```python
from build123d import *

# Parameters (mm, degrees)
SKETCH_1_W          = 100
SKETCH_1_H          = 40
EXTRUDE_1_DEPTH     = 2
EXTRUDE_2_DEPTH     = 2
SKETCH_4_R          = 3.5
CUT_EXTRUDE_1_DEPTH = 2


with BuildPart() as part:
    # 草图1 → 凸台-拉伸1 (new body)
    with BuildSketch(Plane(origin=(0, 0, 0), x_dir=(1, 0, 0), z_dir=(0, 1, 0))):
        with Locations((50, 20)):
            Rectangle(SKETCH_1_W, SKETCH_1_H)
    extrude(amount=EXTRUDE_1_DEPTH)

    # 草图3 → 凸台-拉伸2 (add)
    with BuildSketch(Plane.XY):
        with BuildLine():
            Line((72.5, 0), (27.5, 0))
            Line((27.5, 0), (37.539738947, 55.648838734))
            ThreePointArc((37.539738947, 55.648838734), (35.238312644, 66.663191018), (41.243617117, 76.178906306))
            Line((41.243617117, 76.178906306), (45, 97))
            Line((45, 97), (55, 97))
            Line((55, 97), (58.756382883, 76.178906306))
            ThreePointArc((58.756382883, 76.178906306), (64.761687356, 66.663191018), (62.460261053, 55.648838734))
            Line((62.460261053, 55.648838734), (72.5, 0))
        make_face()
    extrude(amount=EXTRUDE_2_DEPTH)

    # 草图4 → 切除-拉伸1 (cut)
    with BuildSketch(Plane.XY.offset(2)):
        with Locations((50, 64)):
            Circle(SKETCH_4_R)
    extrude(amount=-CUT_EXTRUDE_1_DEPTH, mode=Mode.SUBTRACT)


solid = part.part
```
Build history of the part. All positions in model axes, mm. A direction names the side the tool comes from. Give positions to 0.01 mm unless a question says otherwise; leave off trailing zeros. Loops run counter-clockwise (first coordinate to the right, second up) from the corner with the lowest first, then second, coordinate; pieces in that order, holes last. Notation, with made-up numbers: (66, -23.75) -> (112, -23.75) arc R17 cw to (112, -12.75) -> close; hole circle Ø11 at (62, 89.5). An arc over 180 degrees is marked (long way). One line per question, with ' | ' between items.
Q1. Tool access for faces 4 (the flat face through (50, 40, 0)), 5 (the cylindrical face through (64.732, 66.822, 0.986)): list every direction of +Z, -Z, +X, -X, +Y, -Y with a clear straight run to the whole face (end or side of a thin tool).
Filled sheet:
face 4: -Z, +X, -X, +Y | face 5: +Z, -Z, +X
Q2. Cut at B-B, the plane y = 64. Write the cut outline in (x, z).
Filled sheet:
outline: (35, 0) -> (46.5, 0) -> (46.5, 2) -> (35, 2) -> close; (53.5, 0) -> (65, 0) -> (65, 2) -> (53.5, 2) -> close
Q3. Drill centre lines: line 1 along Y through (x, z) = (50, 0.7); line 2 along Y through (x, z) = (18, -38). Where is each one in solid material? Low to high. Write a range as [from, to].
Filled sheet:
line 1: y = [0, 60.5], [67.5, 97] | line 2: y = [0, 2]
Q4. Cut at A-A, the plane x = 50. Write the cut outline in (y, z).
Filled sheet:
outline: (0, -40) -> (2, -40) -> (2, 0) -> (60.5, 0) -> (60.5, 2) -> (0, 2) -> close; (67.5, 0) -> (97, 0) -> (97, 2) -> (67.5, 2) -> close
Q5. Cut at C-C, the plane z = -34. Write the cut outline in (x, y), plus the area to 3 significant figures.
Filled sheet:
outline: (0, 0) -> (100, 0) -> (100, 2) -> (0, 2) -> close | area: 200 mm²
Q6. Cut at D-D, the plane y = 54. Write the cut outline in (x, z), plus the area to 3 significant figures.
Filled sheet:
outline: (37.24, 0) -> (62.76, 0) -> (62.76, 2) -> (37.24, 2) -> close | area: 51.0 mm²
Q7. Pull direction Y, two halves, no side cores. Call faces 1 (the flat face through (49, 2, -20)), 2 (the flat face through (50, 38, 2)), 3 (the flat face through (32.45, 27.43, 0.99)): pulls with the +Y half, pulls with the -Y half, needs draft (parallel to the pull), parting line crosses it, or undercut.
Filled sheet:
face 1: pulls with the +Y half | face 2: needs draft | face 3: undercut
Q8. Drop flat-ended pins along their axis: pin 1 (3 mm diameter, centred on y = 74, z = -2.5, fed in from +X); pin 2 (12 mm diameter, centred on x = 62, y = 20.5, fed in from -Z); pin 3 (1.5 mm diameter, centred on x = 75, z = -10.5, fed in from +Y); pin 4 (1 mm diameter, centred on x = 9.5, y = 0.5, fed in from +Z). Give the stop position or say it passes through.
Filled sheet:
pin 1: passes through | pin 2: stops at z = 0 | pin 3: stops at y = 2 | pin 4: stops at z = 0
